Check sheet for the modelled part. Datum: model origin and axes. Units: mm. Give positions to 0.01 mm unless a question says otherwise; leave off trailing zeros. Loops run counter-clockwise (first coordinate to the right, second up) from the corner with the lowest first, then second, coordinate; pieces in that order, holes last. Notation, with made-up numbers: (-25.5, 45) - (31.5, 45) arc R19 cw to (31.5, 61) - close; hole circle Ø4 at (37.25, 88). An arc over 180 degrees is marked (long way). Use CSV: the item, a comma, the result in double quotes.
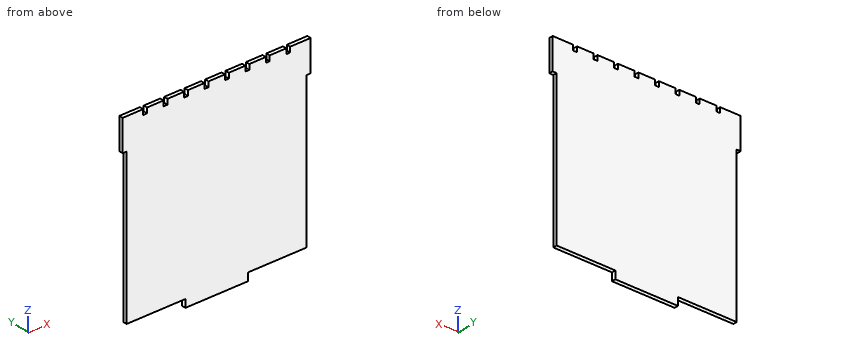
from build123d import *

# Parameters (mm, degrees)
F0_W     = 19.05
F0_H     = 152.4
F0_W_2   = 304.8
F0_H_2   = 38.1
F1_DEPTH = 19.05


with BuildPart() as f1:
    # F0 (on Front) → F1 (new body)
    with BuildSketch(Plane.XZ):
        Polygon((-357.716667, 447.675), (-438.15, 447.675), (-438.15, 295.275), (-438.15, -447.675), (-152.4, -447.675), (152.4, -447.675), (438.15, -447.675), (438.15, 295.275), (438.15, 447.675), (357.716667, 447.675), (357.716667, 422.275), (338.666667, 422.275), (338.666667, 447.675), (258.233333, 447.675), (258.233333, 422.275), (239.183333, 422.275), (239.183333, 447.675), (158.75, 447.675), (158.75, 422.275), (139.7, 422.275), (139.7, 447.675), (59.266667, 447.675), (59.266667, 422.275), (40.216667, 422.275), (40.216667, 447.675), (-40.216667, 447.675), (-40.216667, 422.275), (-59.266667, 422.275), (-59.266667, 447.675), (-139.7, 447.675), (-139.7, 422.275), (-158.75, 422.275), (-158.75, 447.675), (-239.183333, 447.675), (-239.183333, 422.275), (-258.233333, 422.275), (-258.233333, 447.675), (-338.666667, 447.675), (-338.666667, 422.275), (-357.716667, 422.275), align=None)
        with Locations((-447.675, 371.475)):
            Rectangle(F0_W, F0_H)
        with Locations((0, -466.725)):
            Rectangle(F0_W_2, F0_H_2)
        with Locations((447.675, 371.475)):
            Rectangle(F0_W, F0_H)
    extrude(amount=F1_DEPTH)


solid = f1.part
1. Sectioned sample at A-A, the plane z = -261. Record the boundary of the cut face in (x, y), and give its area (3 significant figures).
Completed:
outline,"(-438.15, -19.05) - (438.15, -19.05) - (438.15, 0) - (-438.15, 0) - close"
area,"16,700 mm²"
2. Go/stop test with flat-tipped pins: pin 1 Ø9.5 at (x, y) = (450.5, -7.5) entering from -Z (3 decimals); pin 2 Ø2 at (x, y) = (268.5, -12) entering from -Z (3 decimals); pin 3 Ø9.5 at (x, y) = (-246.5, -11.5) entering from +Z (3 decimals). Record where each tip stops, or that it passes through.
Completed:
pin 1,"stops at z = 295.275"
pin 2,"stops at z = -447.675"
pin 3,"stops at z = 422.275"
3. Scan lines: line 1 along X through (y, z) = (-12, -166); line 2 along Z through (x, y) = (-47, -12) (3 decimals); line 3 along Z through (x, y) = (-176, -4.25) (3 decimals). Record each from-to range of solid material in increasing order.
Completed:
line 1,"x = -438.15 to 438.15"
line 2,"z = -485.775 to 422.275"
line 3,"z = -447.675 to 447.675"
4. Sectioned sample at B-B, the plane x = -212. Record the boundary of the cut face in (y, z) (3 decimals).
Completed:
outline,"(-19.05, -447.675) - (0, -447.675) - (0, 447.675) - (-19.05, 447.675) - close"
